Geometry: final body of the model. Coordinates: model frame, mm. A direction names the side the tool comes from. Coordinates: 2 decimals unless noted, no trailing zeros. Write each loop counter-clockwise with the first axis right and the second up, starting at its lowest first coordinate (ties: lowest second). Pieces come first, ordered by that corner, then holes. Notation, with made-up numbers: (-30.5, -15.5) -> (-20.5, -15.5) arc R16 ccw to (-20.5, 4.5) -> close; hole circle Ø6 at (10.25, 8.5). An arc over 180 degrees is marked (long way). One line per item, written item: value. Start each with the question number.
from build123d import *

# Parameters (mm, degrees)
RESSALTO_EXTRUS_O1_DEPTH = 2.75
ESBO_O4_R                = 1.5
CORTE_EXTRUS_O1_DEPTH    = 56.81185506


with BuildPart() as part:
    # Esboço3 → Ressalto-extrusão1 (new body)
    with BuildSketch(Plane(origin=(0, 0, 0), x_dir=(1, 0, 0), z_dir=(0, 1, 0))):
        with BuildLine():
            Line((-30, 0), (30, 0))
            ThreePointArc((30, 0), (34.716968698, -2.359969453), (35.656560331, -7.55))
            Line((35.656560331, -7.55), (34.321008321, -12.111933867))
            ThreePointArc((34.321008321, -12.111933867), (33.600767374, -13.150604219), (32.401573422, -13.55))
            Line((32.401573422, -13.55), (25.9, -13.55))
            ThreePointArc((25.9, -13.55), (24.485786438, -14.135786438), (23.9, -15.55))
            Line((23.9, -15.55), (23.9, -21.060817198))
            ThreePointArc((23.9, -21.060817198), (23.895174557, -21.199664191), (23.880721513, -21.337841185))
            Line((23.880721513, -21.337841185), (21.140975666, -40.927023988))
            ThreePointArc((21.140975666, -40.927023988), (20.472875962, -42.158981109), (19.160254154, -42.65))
            Line((19.160254154, -42.65), (14.6, -42.65))
            ThreePointArc((14.6, -42.65), (13.185786438, -42.064213562), (12.6, -40.65))
            Line((12.6, -40.65), (12.6, -39.750343786))
            ThreePointArc((12.6, -39.750343786), (12.352304612, -38.786275041), (11.670571453, -38.061001677))
            Line((11.670571453, -38.061001677), (4.490212451, -33.51065789))
            ThreePointArc((4.490212451, -33.51065789), (3.977007924, -33.279233978), (3.419640998, -33.2))
            Line((3.419640998, -33.2), (-3.419640998, -33.2))
            ThreePointArc((-3.419640998, -33.2), (-3.977007924, -33.279233978), (-4.490212451, -33.51065789))
            Line((-4.490212451, -33.51065789), (-11.670571453, -38.061001677))
            ThreePointArc((-11.670571453, -38.061001677), (-12.352304612, -38.786275041), (-12.6, -39.750343786))
            Line((-12.6, -39.750343786), (-12.6, -40.65))
            ThreePointArc((-12.6, -40.65), (-13.185786438, -42.064213562), (-14.6, -42.65))
            Line((-14.6, -42.65), (-19.160254154, -42.65))
            ThreePointArc((-19.160254154, -42.65), (-20.472875962, -42.158981109), (-21.140975666, -40.927023988))
            Line((-21.140975666, -40.927023988), (-23.880721513, -21.337841185))
            ThreePointArc((-23.880721513, -21.337841185), (-23.895174557, -21.199664191), (-23.9, -21.060817198))
            Line((-23.9, -21.060817198), (-23.9, -15.55))
            ThreePointArc((-23.9, -15.55), (-24.485786438, -14.135786438), (-25.9, -13.55))
            Line((-25.9, -13.55), (-32.401573422, -13.55))
            ThreePointArc((-32.401573422, -13.55), (-33.600767374, -13.150604219), (-34.321008321, -12.111933867))
            Line((-34.321008321, -12.111933867), (-35.656560331, -7.55))
            ThreePointArc((-35.656560331, -7.55), (-34.716968698, -2.359969453), (-30, 0))
        make_face()
    extrude(amount=RESSALTO_EXTRUS_O1_DEPTH)

    # Esboço4 → Corte-extrusão1 (cut, through all)
    with BuildSketch(Plane(origin=(0, 2.75, 0), x_dir=(1, 0, 0), z_dir=(0, 1, 0))):
        with Locations(Location((3.5, -5.893985085, 0), (0, 0, 270))):
            Circle(ESBO_O4_R)
        with Locations(Location((30, -5.893985085, 0), (0, 0, 270))):
            Circle(ESBO_O4_R)
        with Locations(Location((19.9, -4.95, 0), (0, 0, 270))):
            Circle(ESBO_O4_R)
        with Locations(Location((19.9, -18.45, 0), (0, 0, 270))):
            Circle(ESBO_O4_R)
        with Locations(Location((17.1, -38.65, 0), (0, 0, 270))):
            Circle(ESBO_O4_R)
        with Locations(Location((-3.5, -5.893985085, 0), (0, 0, 90))):
            Circle(ESBO_O4_R)
        with Locations(Location((-17.1, -38.65, 0), (0, 0, 90))):
            Circle(ESBO_O4_R)
        with Locations(Location((-19.9, -18.45, 0), (0, 0, 90))):
            Circle(ESBO_O4_R)
        with Locations(Location((-19.9, -4.95, 0), (0, 0, 90))):
            Circle(ESBO_O4_R)
        with Locations(Location((-30, -5.893985085, 0), (0, 0, 90))):
            Circle(ESBO_O4_R)
        with BuildLine():
            Line((3.5, -25.229610701), (3.5, -15.814435009))
            ThreePointArc((3.5, -15.814435009), (4.187027668, -14.864672766), (5.304096639, -15.219936401))
            Line((5.304096639, -15.219936401), (10.25973036, -21.922741689))
            ThreePointArc((10.25973036, -21.922741689), (10.405395965, -22.204267965), (10.455633721, -22.517240297))
            Line((10.455633721, -22.517240297), (10.455633721, -28.370099513))
            ThreePointArc((10.455633721, -28.370099513), (9.937668094, -29.246251819), (8.920347995, -29.214770568))
            Line((8.920347995, -29.214770568), (3.964714273, -26.074281756))
            ThreePointArc((3.964714273, -26.074281756), (3.623847694, -25.711645074), (3.5, -25.229610701))
        make_face()
        with BuildLine():
            Line((-8.920347995, -29.214770568), (-3.964714273, -26.074281756))
            ThreePointArc((-3.964714273, -26.074281756), (-3.623847694, -25.711645074), (-3.5, -25.229610701))
            Line((-3.5, -25.229610701), (-3.5, -15.814435009))
            ThreePointArc((-3.5, -15.814435009), (-4.187027668, -14.864672766), (-5.304096639, -15.219936401))
            Line((-5.304096639, -15.219936401), (-10.25973036, -21.922741689))
            ThreePointArc((-10.25973036, -21.922741689), (-10.405395965, -22.204267965), (-10.455633721, -22.517240297))
            Line((-10.455633721, -22.517240297), (-10.455633721, -28.370099513))
            ThreePointArc((-10.455633721, -28.370099513), (-9.937668094, -29.246251819), (-8.920347995, -29.214770568))
        make_face()
    extrude(amount=-CORTE_EXTRUS_O1_DEPTH, mode=Mode.SUBTRACT)


solid = part.part
Q1. Access query for faces 4 (the cylindrical face through (9.95, 1.39, 29.24)), 5 (the flat face through (23.9, 1, 18)), 6 (the flat face through (-23.9, 1, 18)), 7 (the cylindrical face through (-12.345, 1.356, 38.774)). Directions: +Z, -Z, +X, -X, +Y, -Y. A direction counts if a zero-diameter tool reaches every point of the face in a straight line with its end or side. Return the directions, or none.
Q2. Cut plane A-A on x = -17.1. Output: boundary loops of the cut face in (y, z), and give its area (3 significant figures).
Q3. Line query: L1, parallel to Z at x = 19, y = 1.95; L2, parallel to X at y = 0.9, z = 38.65; L3, parallel to Z at x = -17.1, y = 1.25. Output: solid intervals per line, ascending. Write a range as from..to.
Q4. Cut plane B-B on x = 19.9. Output: boundary loops of the cut face in (y, z), and give its area (3 significant figures).
Q5. Cut plane D-D on z = 18.45. Output: boundary loops of the cut face in (x, y), and give its area (3 significant figures).
Q6. Cut plane C-C on z = 24. Output: boundary loops of the cut face in (x, y), and give its area (3 significant figures).
Q7. Draft query along Z for faces 1 (the cylindrical face through (-2.587, 1.394, 7.084)), 2 (the flat face through (1, 0, 16)), 3 (the cylindrical face through (20.488, 1.356, 42.146)). Return one class per face: pulls with the +Z half, pulls with the -Z half, needs draft (parallel to the pull), parting line crosses it, or undercut.
Q8. First-contact query: P1, Ø1.4, axis at y = 2, z = 19.5, coming from the +X side; P2, Ø1.5, axis at y = 1, z = 11.5, coming from the -X side; P3, Ø1, axis at y = 1, z = 40, coming from the -X side; P4, Ø2, axis at x = -7.5, z = 21, coming from the +Y side. Flat tips, straight axial feed; report the tip coordinate or a pass-through.
Solution:
1. face 4: +Y, -Y
1. face 5: +Z, +X, +Y, -Y
1. face 6: +Z, -X, +Y, -Y
1. face 7: +Z, +Y, -Y
2. outline: (0, 0) -> (2.75, 0) -> (2.75, 37.15) -> (0, 37.15) -> close; (0, 40.15) -> (2.75, 40.15) -> (2.75, 42.65) -> (0, 42.65) -> close
2. area: 109 mm²
3. L1: 0..3.75, 6.15..17.25, 19.65..42.65
3. L2: -21.46..-18.6, -15.6..-12.27, 12.27..15.6, 18.6..21.46
3. L3: 0..37.15, 40.15..42.65
4. outline: (0, 0) -> (2.75, 0) -> (2.75, 3.45) -> (0, 3.45) -> close; (0, 6.45) -> (2.75, 6.45) -> (2.75, 16.95) -> (0, 16.95) -> close; (0, 19.95) -> (2.75, 19.95) -> (2.75, 42.51) -> (0, 42.51) -> close
4. area: 100 mm²
5. outline: (-23.9, 0) -> (-21.4, 0) -> (-21.4, 2.75) -> (-23.9, 2.75) -> close; (-18.4, 0) -> (-7.69, 0) -> (-7.69, 2.75) -> (-18.4, 2.75) -> close; (-3.5, 0) -> (3.5, 0) -> (3.5, 2.75) -> (-3.5, 2.75) -> close; (7.69, 0) -> (18.4, 0) -> (18.4, 2.75) -> (7.69, 2.75) -> close; (21.4, 0) -> (23.9, 0) -> (23.9, 2.75) -> (21.4, 2.75) -> close
5. area: 91.9 mm²
6. outline: (-23.51, 0) -> (-10.46, 0) -> (-10.46, 2.75) -> (-23.51, 2.75) -> close; (-3.5, 0) -> (3.5, 0) -> (3.5, 2.75) -> (-3.5, 2.75) -> close; (10.46, 0) -> (23.51, 0) -> (23.51, 2.75) -> (10.46, 2.75) -> close
6. area: 91.0 mm²
7. face 1: undercut
7. face 2: needs draft
7. face 3: pulls with the +Z half
8. P1: x = 23.9
8. P2: x = -34.72
8. P3: x = -21.34
8. P4: through
